```python
from build123d import *

# Parameters (mm, degrees)
BOSS_EXTRUDE1_DEPTH = 2.5
BOSS_EXTRUDE2_DEPTH = 2.5
BOSS_EXTRUDE2_TAPER = 25
SKETCH4_R           = 2.5
CUT_EXTRUDE1_DEPTH  = 90.131924696


with BuildPart() as part:
    # Sketch1 → Boss-Extrude1 (new body)
    with BuildSketch(Plane.XY):
        with BuildLine():
            Line((-46.5, 57.094220373), (-46.5, 48.094220373))
            ThreePointArc((-46.5, 48.094220373), (-42.572396728, 44.094875587), (-38.502620643, 47.949450635))
            ThreePointArc((-38.502620643, 47.949450635), (-36.387640055, 50.707965196), (-33.087155105, 49.617394443))
            ThreePointArc((-33.087155105, 49.617394443), (-22.211018918, 43.548965481), (-10.5, 47.787857357))
            ThreePointArc((-10.5, 47.787857357), (0, 52.075714714), (10.5, 47.787857357))
            ThreePointArc((10.5, 47.787857357), (22.211018918, 43.548965481), (33.087155105, 49.617394443))
            ThreePointArc((33.087155105, 49.617394443), (36.387640055, 50.707965196), (38.502620643, 47.949450635))
            ThreePointArc((38.502620643, 47.949450635), (42.572396728, 44.094875587), (46.5, 48.094220373))
            Line((46.5, 48.094220373), (46.5, 57.094220373))
            ThreePointArc((46.5, 57.094220373), (45.830505203, 59.848437918), (43.971428571, 61.988010691))
            ThreePointArc((43.971428571, 61.988010691), (0, 76), (-43.971428571, 61.988010691))
            ThreePointArc((-43.971428571, 61.988010691), (-45.830505203, 59.848437918), (-46.5, 57.094220373))
        make_face()
    extrude(amount=BOSS_EXTRUDE1_DEPTH)

    # Sketch3 → Boss-Extrude2 (add)
    with BuildSketch(Plane.XY.offset(2.5)):
        with BuildLine():
            ThreePointArc((24.71651229, 68.853141378), (0, 73.155048065), (-24.71651229, 68.853141378))
            ThreePointArc((-24.71651229, 68.853141378), (-30.319675299, 52.656743004), (-13.3, 50.644428729))
            ThreePointArc((-13.3, 50.644428729), (0, 56.075714714), (13.3, 50.644428729))
            ThreePointArc((13.3, 50.644428729), (30.319675299, 52.656743004), (24.71651229, 68.853141378))
        make_face()
    extrude(amount=BOSS_EXTRUDE2_DEPTH, taper=BOSS_EXTRUDE2_TAPER)

    # Sketch4 → Cut-Extrude1 (cut, through all)
    with BuildSketch(Plane.XY.offset(2.5)):
        with Locations((-42.5, 48.094220373)):
            Circle(SKETCH4_R)
        with Locations((42.5, 48.094220373)):
            Circle(SKETCH4_R)
    extrude(amount=-CUT_EXTRUDE1_DEPTH, mode=Mode.SUBTRACT)


solid = part.part
```
The listing builds one solid part. Answer for the finished solid, in the listing's coordinates (mm). A direction names the side the tool comes from. Coordinates: 2 decimals unless noted, no trailing zeros. Loops run counter-clockwise (first coordinate to the right, second up) from the corner with the lowest first, then second, coordinate; pieces in that order, holes last. Notation, with made-up numbers: (-6.75, 13.5) - (33.25, 13.5) arc R12 cw to (33.25, 18.5) - close; hole circle Ø4 at (-12.5, 41.25). An arc over 180 degrees is marked (long way). Use a Markdown table: item, result. Add a question column.
1) The part is cut by section A-A, the plane x = -42.5. Give the vertices of the cut face in (y, z).
2) The mould has two halves that part along Y. Classify faces 1 (the cylindrical face through (42.485, 44.094, 1.232)), 2 (the flat face through (46.5, 53, 1)), 3 (the cylindrical face through (-41.156, 50.202, 1.268)), 4 (the cylindrical face through (43.844, 50.202, 1.268)): released by +Y, released by -Y, zero draft, split by the parting line, or undercut.
3) Find the intervals of material crossed by line 1 (X direction, y = 49.5, z = 1.8); line 2 (X direction, y = 47, z = 1.5); line 3 (Z direction, x = -32, y = 61), in increasing order.
4) The part is cut by section C-C, the plane z = 3.9. Give the vertices of the cut face in (x, y), and give its area (3 significant figures).
5) Given pin 1 (4 mm diameter, centred on x = -42.5, y = 48.09, fed in from +Z); pin 2 (1.5 mm diameter, centred on x = -28.5, z = 3.5, fed in from +Y) (3 decimals), each flat-ended and moving along its own axis, determine where each tip first touches the part or whether it passes through.
6) The part is cut by section B-B, the plane y = 58.5. Give the vertices of the cut face in (x, z), and give its area (3 significant figures).
7) For faces 5 (the flat face through (0, 54, 2.5)), 6 (the cylindrical face through (45.85, 59.81, 1.23)), determine the directions among +Z, -Z, +X, -X, +Y, -Y from which every point of the face is accessible in a straight line to the end or side of a thin tool.
Here are the results:
| question | item | result |
|---|---|---|
| 1 | outline | (44.09, 0) - (45.59, 0) - (45.59, 2.5) - (44.09, 2.5) - close; (50.59, 0) - (63.01, 0) - (63.01, 2.5) - (50.59, 2.5) - close |
| 2 | face 1 | released by -Y |
| 2 | face 2 | zero draft |
| 2 | face 3 | undercut |
| 2 | face 4 | undercut |
| 3 | line 1 | x = -46.5 to -44.57, -40.43 to -38, -33 to -8.4, 8.4 to 33, 38 to 40.43, 44.57 to 46.5 |
| 3 | line 2 | x = -46.35 to -44.75, -40.25 to -38.65, -30.63 to -11.37, 11.37 to 30.63, 38.65 to 40.25, 44.75 to 46.35 |
| 3 | line 3 | z = 0 to 2.5 |
| 4 | outline | (-24.5, 68.24) arc R10.35 ccw (long way) to (-13.76, 51.11) arc R19.65 cw to (13.76, 51.11) arc R10.35 ccw (long way) to (24.5, 68.24) arc R72.5 ccw to start |
| 4 | area | 1,120 mm^2 |
| 5 | pin 1 | passes through |
| 5 | pin 2 | stops at y = 66.735 |
| 6 | outline | (-46.33, 0) - (46.33, 0) - (46.33, 2.5) - (32, 2.5) - (30.83, 5) - (-30.83, 5) - (-32, 2.5) - (-46.33, 2.5) - close |
| 6 | area | 389 mm^2 |
| 7 | face 5 | +Z |
| 7 | face 6 | +Z, -Z, +X, +Y |
